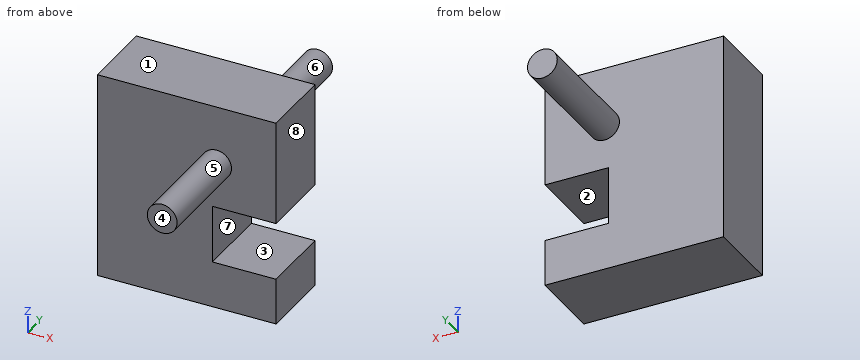
```python
from build123d import *

# Parameters (mm, degrees)
F1_DEPTH      = 25
F2_R          = 5
F3_DEPTH      = 60
F3_DEPTH_BACK = 40


with BuildPart() as f1:
    # F0 (on Front) → F1 (new body)
    with BuildSketch(Plane.XZ):
        Polygon((0, 83.9650441706), (-60, 83.9650441706), (-60, 13.9650441706), (0, 13.9650441706), (0, 29.5586726815), (-21.3913675398, 29.5586726815), (-21.3913675398, 48.9650441706), (0, 48.9650441706), align=None)
    extrude(amount=F1_DEPTH)

    # F2 (on face) → F3 (join, two sides)
    with BuildSketch(Plane(origin=(0, 0, 0), x_dir=(-1, 0, 0), z_dir=(0, 1, 0))) as f3_sk:
        with Locations((20, 63.9650441706)):
            Circle(F2_R)
    extrude(amount=-F3_DEPTH)
    extrude(f3_sk.sketch, amount=F3_DEPTH_BACK)


solid = f1.part
```
CAD build for the part. Positions are in the model's coordinates, mm. Face numbers are marked on the shaded views. A direction names the side the tool comes from. Round coordinates to 2 decimals unless told otherwise and drop trailing zeros. Write each loop counter-clockwise with the first axis right and the second up, starting at its lowest first coordinate (ties: lowest second). Pieces come first, ordered by that corner, then holes. Notation, with made-up numbers: (20.5, 35.25) -> (36.5, 35.25) arc R26 cw to (36.5, 69.25) -> close; hole circle Ø10 at (-17, 20). An arc over 180 degrees is marked (long way). Answer in a Markdown table with one row per item. Add a question column.
Item 1: Drill centre lines: line 1 (Y direction, x = -43, z = 23); line 2 (Z direction, x = -13, y = -20.5); line 3 (X direction, y = -12, z = 35). Where is each one in solid material? Low to high. Write a range as from..to.
Item 2: Saw through at C-C, the plane x = -37.5. Write the cut outline in (y, z).
Item 3: Saw through at A-A, the plane x = -20. Write the cut outline in (y, z).
Item 4: Mould opens along Z. For the marked faces 1, 2, 3 and 4 say: pulls with the +Z half, pulls with the -Z half, needs draft (parallel to the pull), parting line crosses it, or undercut.
Item 5: Saw through at B-B, the plane z = 71. Write the cut outline in (x, y).
Item 6: Drop flat-ended pins along their axis: pin 1 Ø1.5 at (y, z) = (-7, 24) entering from +X; pin 2 Ø15.5 at (y, z) = (-10, 40.5) entering from +X; pin 3 Ø3 at (x, z) = (-8.5, 28) entering from -Y; pin 4 Ø8 at (y, z) = (26, 67.5) entering from -X. Give the stop position or say it passes through.
Item 7: Which spindle directions (+Z, -Z, +X, -X, +Y, -Y) get a long thin tool onto all of the face, cutting with end or side? Do the marked faces 5, 6, 7 and 8. Say none if no direction does.
Item 8: Saw through at D-D, the plane y = -49.5. Write the cut outline in (x, z).
Findings below:
| question | item | result |
|---|---|---|
| 1 | line 1 | y = -25..0 |
| 1 | line 2 | z = 13.97..29.56, 48.97..83.97 |
| 1 | line 3 | x = -60..-21.39 |
| 2 | outline | (-25, 13.97) -> (0, 13.97) -> (0, 83.97) -> (-25, 83.97) -> close |
| 3 | outline | (-60, 58.97) -> (-25, 58.97) -> (-25, 48.97) -> (0, 48.97) -> (0, 58.97) -> (40, 58.97) -> (40, 68.97) -> (0, 68.97) -> (0, 83.97) -> (-25, 83.97) -> (-25, 68.97) -> (-60, 68.97) -> close; (-25, 13.97) -> (0, 13.97) -> (0, 29.56) -> (-25, 29.56) -> close |
| 4 | face 1 | pulls with the +Z half |
| 4 | face 2 | undercut |
| 4 | face 3 | undercut |
| 4 | face 4 | needs draft |
| 5 | outline | (-60, -25) -> (0, -25) -> (0, 0) -> (-60, 0) -> close |
| 6 | pin 1 | stops at x = 0 |
| 6 | pin 2 | stops at x = -21.39 |
| 6 | pin 3 | stops at y = -25 |
| 6 | pin 4 | stops at x = -25 |
| 7 | face 5 | -Y |
| 7 | face 6 | +Y |
| 7 | face 7 | +X, +Y, -Y |
| 7 | face 8 | +Z, -Z, +X, +Y, -Y |
| 8 | outline | circle Ø10 at (-20, 63.97) |
